Drawing for the job (mm, zero at the part's lowest x, y, z). Give positions to 0.01 mm unless a question says otherwise; leave off trailing zeros. Write each loop counter-clockwise with the first axis right and the second up, starting at its lowest first coordinate (ties: lowest second). Pieces come first, ordered by that corner, then holes. Notation, with made-up numbers: M 29,62 L 36,62 A7 cw 36,75 Z; hole C -37,2.5 d1. An arc over 180 degrees is marked long. Answer as a JSON object with one key per item and string values. Group by question number.
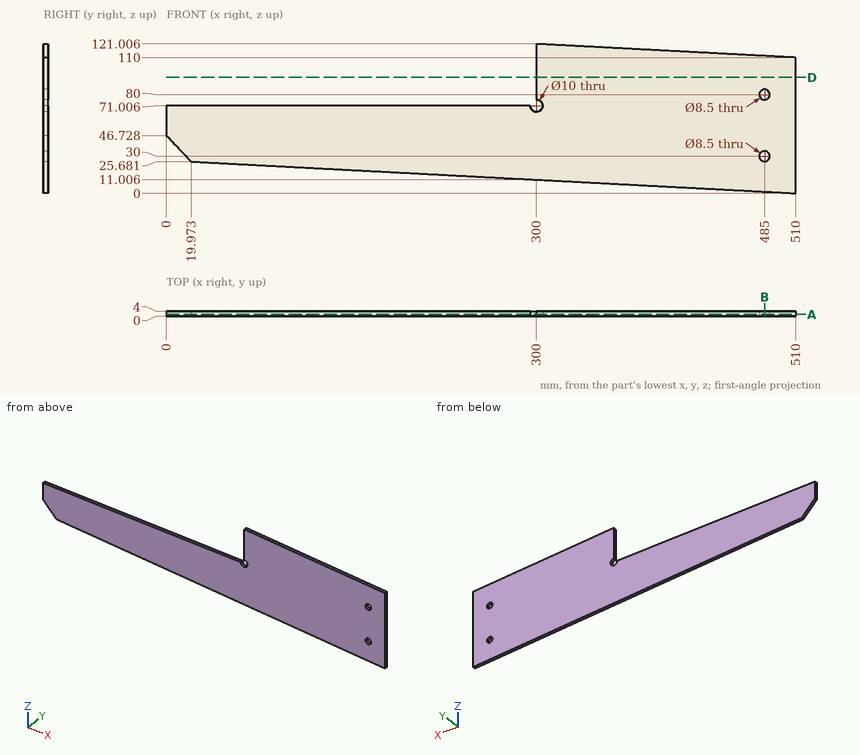
Q1. Slice it at B-B, the plane x = 485. Write the cut outline in (y, z).
Q2. Slice it at A-A, the plane y = 1.4. Count the separate pieces of the cut face and the enclosed holes in it, then the cut area to 3 significant figures.
Q3. Wall check: L1, parallel to Z at x = 485, y = 1.45; L2, parallel to X at y = 2.3, z = 109; L3, parallel to X at y = 2.9, z = 83. Give the ranges that are in metal, low to high.
Q4. Drop flat-ended pins along their axis: P1, Ø1.5, axis at y = 2.5, z = 73, coming from the -X side; P2, Ø1.2, axis at x = 103, y = 2.5, coming from the +Z side; P3, Ø1.5, axis at x = 209.5, y = 2, coming from the -Z side. Give the stop position or say it passes through.
Q5. Slice it at D-D, the plane z = 94. Write the cut outline in (x, y), then the cut area to 3 significant figures.
Solved:
{
 "1": {"outline": "M 0,1.31 L 4,1.31 L 4,25.75 L 0,25.75 Z; M 0,34.25 L 4,34.25 L 4,75.75 L 0,75.75 Z; M 0,84.25 L 4,84.25 L 4,111.31 L 0,111.31 Z"},
 "2": {"separate pieces": "1", "enclosed holes": "2", "area": "38,400 mm²"},
 "3": {"L1": "z = 1.31 to 25.75, 34.25 to 75.75, 84.25 to 111.31", "L2": "x = 300 to 510", "L3": "x = 300 to 481.99, 488.01 to 510"},
 "4": {"P1": "stops at x = 304.18", "P2": "stops at z = 71.01", "P3": "stops at z = 15.71"},
 "5": {"outline": "M 300,0 L 510,0 L 510,4 L 300,4 Z", "area": "840 mm²"}
}
